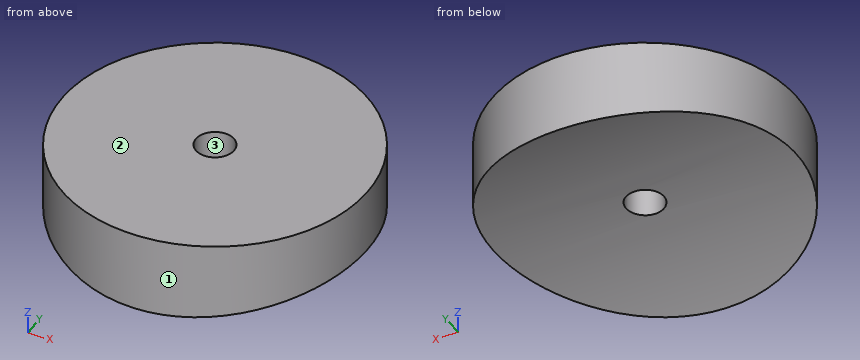
from build123d import *

# Parameters (mm, degrees)
F0_R     = 12
F1_DEPTH = 5
F2_R     = 53.4
F3_DEPTH = 12.5
F4_R     = 1.5
F5_DEPTH = 6.366781


with BuildPart() as f1:
    # F0 (on Top) → F1 (new body, symmetric)
    with BuildSketch(Plane.XY):
        Circle(F0_R)
    extrude(amount=F1_DEPTH, both=True)

    # F2 (on Right) → F3 (cut, symmetric)
    with BuildSketch(Plane.YZ):
        with Locations((0, -53.4)):
            Circle(F2_R)
    extrude(amount=F3_DEPTH, both=True, mode=Mode.SUBTRACT)

    # F4 (on face) → F5 (cut, through all)
    with BuildSketch(Plane.XY.offset(5)):
        Circle(F4_R)
    extrude(amount=-F5_DEPTH, mode=Mode.SUBTRACT)


solid = f1.part
Can you work these out from the model? Positions are in its coordinate system, mm. Face numbers are marked on the shaded views. Give positions to 0.01 mm unless a question says otherwise; leave off trailing zeros. Write each loop counter-clockwise with the first axis right and the second up, starting at its lowest first coordinate (ties: lowest second). Pieces come first, ordered by that corner, then holes. Notation, with made-up numbers: (16.5, 36.5) -> (72.5, 36.5) arc R11 ccw to (72.5, 53.5) -> close; hole circle Ø2 at (-39, -3). An arc over 180 degrees is marked (long way). Answer as a JSON object with one key per item and string values. Group by question number.
Item 1: Please list where these lines run through material, in increasing order: line 1 (Y direction, x = 0, z = 2.3); line 2 (Z direction, x = -10, y = 1.75). Write a range as [from, to].
Item 2: We'd pull the mould along Y, two halves only. Please class the marked faces 1, 2 and 3: +Y half, -Y half, draft (parallel to the pull), parting line (faces both ways), or undercut.
Item 3: Suppose I cut it at C-C (z = 2.25). Please give me the cut outline in (x, y).
Item 4: Suppose I cut it at A-A (x = 0). Please give me the cut outline in (y, z).
Item 5: Suppose I cut it at B-B (y = 0). Please give me the cut outline in (x, z), plus the area to 3 significant figures.
Item 6: Suppose I cut it at D-D (y = 2.5). Please give me the cut outline in (x, z).
Item 7: I'm going to push flat-ended pins straight in: P1, Ø3, axis at x = -2.5, z = 4, coming from the -Y side; P2, Ø5, axis at x = 6.5, y = 0.5, coming from the -Z side; P3, Ø4, axis at x = 0, y = 0, coming from the -Z side. Where does each tip first touch, or does it pass through?
Findings:
{
 "1": {"line 1": "y = [-12, -1.5], [1.5, 12]", "line 2": "z = [-0.03, 5]"},
 "2": {"face 1": "parting line", "face 2": "draft", "face 3": "undercut"},
 "3": {"outline": "circle Ø24 at (0, 0); hole circle Ø3 at (0, 0)"},
 "4": {"outline": "(-12, -1.37) arc R53.4 cw to (-1.5, -0.02) -> (-1.5, 5) -> (-12, 5) -> close; (1.5, -0.02) arc R53.4 cw to (12, -1.37) -> (12, 5) -> (1.5, 5) -> close"},
 "5": {"outline": "(-12, 0) -> (-1.5, 0) -> (-1.5, 5) -> (-12, 5) -> close; (1.5, 0) -> (12, 0) -> (12, 5) -> (1.5, 5) -> close", "area": "105 mm²"},
 "6": {"outline": "(-11.74, -0.06) -> (11.74, -0.06) -> (11.74, 5) -> (-11.74, 5) -> close"},
 "7": {"P1": "stops at y = -11.96", "P2": "stops at z = -0.08", "P3": "stops at z = -0.04"}
}
